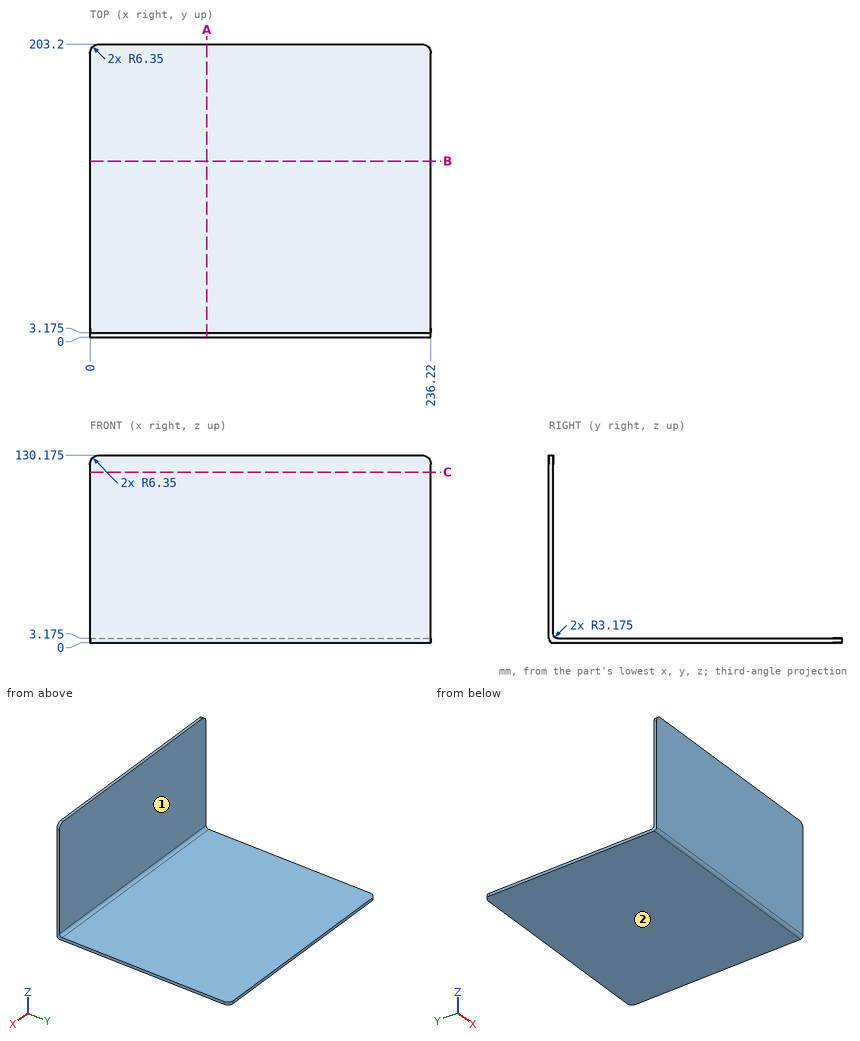
Study the drawing (mm; zero at the part's minimum x, y, z) and answer. A direction names the side the tool comes from. Give positions to 0.01 mm unless a question says otherwise; leave off trailing zeros. Order: outer loops, then holes, each group sorted by start corner. A loop starts at its lowest first (then second) coordinate and runs counter-clockwise, first axis right, second up. Notation, with made-up numbers: (9, -30.5) - (48, -30.5) arc R26 cw to (48, -4.5) - close; hole circle Ø7 at (-22.75, 19.25). An arc over 180 degrees is marked (long way). Answer in a Markdown table with one row per item. Add a question column.
Q1. The part is cut by section A-A (x = 81). Determine the outline of the cut face in (y, z) (3 decimals), then the cut area to 3 significant figures.
Q2. Find the intervals of material crossed by line 1 along Y through (x, z) = (11.5, 43.5) (3 decimals), in increasing order. Write a range as [from, to].
Q3. Given P1, Ø1, axis at x = 112.5, z = 54.5, coming from the +Y side (3 decimals); P2, Ø3, axis at x = 103.5, y = 26.5, coming from the +Z side (3 decimals), each flat-ended and moving along its own axis, determine where each tip first touches the part or whether it passes through.
Q4. Which of the six approach directions +Z, -Z, +X, -X, +Y, -Y give full straight-line access (tool end or side, diameter ignored) to the marked faces 1 and 2?
Q5. The part is cut by section B-B (y = 122). Determine the outline of the cut face in (x, z) (3 decimals).
Determined:
| question | item | result |
|---|---|---|
| 1 | outline | (0, 3.175) arc R3.175 ccw to (3.175, 0) - (203.2, 0) - (203.2, 3.175) - (6.35, 3.175) arc R3.175 cw to (3.175, 6.35) - (3.175, 130.175) - (0, 130.175) - close |
| 1 | area | 1,050 mm² |
| 2 | line 1 | y = [0, 3.175] |
| 3 | P1 | stops at y = 3.175 |
| 3 | P2 | stops at z = 3.175 |
| 4 | face 1 | +Z, +X, -X, +Y |
| 4 | face 2 | -Z, +X, -X, +Y, -Y |
| 5 | outline | (0, 0) - (236.22, 0) - (236.22, 3.175) - (0, 3.175) - close |
